Check sheet for the modelled part. Datum: model origin and axes. Units: mm. A direction names the side the tool comes from. Round coordinates to 2 decimals unless told otherwise and drop trailing zeros. Loops run counter-clockwise (first coordinate to the right, second up) from the corner with the lowest first, then second, coordinate; pieces in that order, holes last. Notation, with made-up numbers: (18, 27.5) - (52, 27.5) arc R19 ccw to (52, 44.5) - close; hole circle Ø6 at (-27.5, -11). An arc over 180 degrees is marked (long way). Return JSON: item names as keys, results as strings.
from build123d import *

# Parameters (mm, degrees)
SKETCH1_R           = 41
BOSS_EXTRUDE1_DEPTH = 6
BOSS_EXTRUDE2_DEPTH = 8
BOSS_EXTRUDE3_DEPTH = 7
SKETCH4_W           = 40.6
SKETCH4_H           = 20.7
CUT_EXTRUDE1_DEPTH  = 7
SKETCH5_R           = 9.55
CUT_EXTRUDE2_DEPTH  = 6.2
SKETCH6_R           = 7
CUT_EXTRUDE3_DEPTH  = 8
SKETCH7_R           = 11
SKETCH7_R_2         = 1.7
CUT_EXTRUDE4_DEPTH  = 6
SKETCH8_R           = 3.25
CUT_EXTRUDE6_DEPTH  = 3.3
SKETCH10_R          = 2.1
CUT_EXTRUDE8_DEPTH  = 5.5
FILLET1_R           = 3
CHAMFER1_SIZE       = 0.8
SKETCH11_W          = 7.2
SKETCH11_H          = 2
CUT_EXTRUDE9_DEPTH  = 2


with BuildPart() as part:
    # Sketch1 → Boss-Extrude1 (new body)
    with BuildSketch(Plane(origin=(0, 0, 0), x_dir=(1, 0, 0), z_dir=(0, 1, 0))):
        with Locations(Location((0, 0, 0), (0, 0, 270))):
            Circle(SKETCH1_R)
    extrude(amount=BOSS_EXTRUDE1_DEPTH)

    # Sketch2 → Boss-Extrude2 (add)
    with BuildSketch(Plane.XY.offset(-30)):
        with BuildLine():
            Line((-24, 0), (24, 0))
            Line((24, 0), (15.461253, 32.066997))
            ThreePointArc((15.461253, 32.066997), (0, 43.95000027), (-15.461253, 32.066997))
            Line((-15.461253, 32.066997), (-24, 0))
        make_face()
    extrude(amount=BOSS_EXTRUDE2_DEPTH)

    # Sketch3 → Boss-Extrude3 (add)
    with BuildSketch(Plane.XY.offset(22)):
        with BuildLine():
            Line((-40, 0), (20, 0))
            Line((20, 0), (20, 33))
            ThreePointArc((20, 33), (17.071067812, 40.071067812), (10, 43))
            Line((10, 43), (-30, 43))
            ThreePointArc((-30, 43), (-37.071067812, 40.071067812), (-40, 33))
            Line((-40, 33), (-40, 0))
        make_face()
    extrude(amount=BOSS_EXTRUDE3_DEPTH)

    # Sketch4 → Cut-Extrude1 (cut)
    with BuildSketch(Plane.XY.offset(22)):
        with Locations((-10.1, 28.05)):
            Rectangle(SKETCH4_W, SKETCH4_H)
    extrude(amount=CUT_EXTRUDE1_DEPTH, mode=Mode.SUBTRACT)

    # Sketch5 → Cut-Extrude2 (cut)
    with BuildSketch(Plane.XY.offset(-30)):
        with Locations(Location((0, 27.95, 0), (0, 0, 180))):
            Circle(SKETCH5_R)
    extrude(amount=CUT_EXTRUDE2_DEPTH, mode=Mode.SUBTRACT)

    # Sketch6 → Cut-Extrude3 (cut)
    with BuildSketch(Plane.XY.offset(-30)):
        with Locations((0, 27.95)):
            Circle(SKETCH6_R)
    extrude(amount=CUT_EXTRUDE3_DEPTH, mode=Mode.SUBTRACT)

    # Sketch7 → Cut-Extrude4 (cut)
    with BuildSketch(Plane(origin=(0, 0, 0), x_dir=(1, 0, 0), z_dir=(0, 1, 0))):
        with Locations(Location((0, 0, 0), (0, 0, 270))):
            Circle(SKETCH7_R)
        with Locations(Location((30, 15, 0), (0, 0, 270))):
            Circle(SKETCH7_R_2)
        with Locations(Location((30, -15, 0), (0, 0, 270))):
            Circle(SKETCH7_R_2)
        with Locations(Location((-30, 15, 0), (0, 0, 270))):
            Circle(SKETCH7_R_2)
        with Locations(Location((-30, -15, 0), (0, 0, 270))):
            Circle(SKETCH7_R_2)
    extrude(amount=CUT_EXTRUDE4_DEPTH, mode=Mode.SUBTRACT)

    # Sketch8 → Cut-Extrude6 (cut)
    with BuildSketch(Plane(origin=(0, 6, 0), x_dir=(1, 0, 0), z_dir=(0, 1, 0))):
        with Locations(Location((30, 15, 0), (0, 0, 270))):
            Circle(SKETCH8_R)
        with Locations(Location((30, -15, 0), (0, 0, 270))):
            Circle(SKETCH8_R)
        with Locations(Location((-30, 15, 0), (0, 0, 270))):
            Circle(SKETCH8_R)
        with Locations(Location((-30, -15, 0), (0, 0, 270))):
            Circle(SKETCH8_R)
    extrude(amount=-CUT_EXTRUDE6_DEPTH, mode=Mode.SUBTRACT)

    # Sketch10 → Cut-Extrude8 (cut)
    with BuildSketch(Plane.XY.offset(29)):
        with Locations((-34.811, 23.025)):
            Circle(SKETCH10_R)
        with Locations((-34.811, 32.875)):
            Circle(SKETCH10_R)
        with Locations((14.611, 23.025)):
            Circle(SKETCH10_R)
        with Locations((14.611, 32.875)):
            Circle(SKETCH10_R)
    extrude(amount=-CUT_EXTRUDE8_DEPTH, mode=Mode.SUBTRACT)

    # Fillet1
    fillet1_edges = [part.edges().sort_by_distance(p)[0] for p in [
        (0, 6, -22),
        (-7.298843892, 6, 22),
    ]]
    fillet(fillet1_edges, radius=FILLET1_R)

    # Chamfer1
    chamfer1_edges = [part.edges().sort_by_distance(p)[0] for p in [
        (-30, 0, 13.3),
        (-30, 0, -16.7),
        (30, 0, 13.3),
        (30, 0, -16.7),
    ]]
    chamfer(chamfer1_edges, length=CHAMFER1_SIZE)

    # Sketch11 → Cut-Extrude9 (cut)
    with BuildSketch(Plane.XY.offset(29)):
        with Locations((-33.8, 27.95)):
            Rectangle(SKETCH11_W, SKETCH11_H)
        with Locations((13.6, 27.95)):
            Rectangle(SKETCH11_W, SKETCH11_H)
    extrude(amount=-CUT_EXTRUDE9_DEPTH, mode=Mode.SUBTRACT)


solid = part.part
Q1. Draft check along X on faces 5 (the face through (17.15, 39.99, 25.45)), 6 (the face through (9, 0, 9)), 7 (the face through (26.827, 4.373, -15.705)). Enter one of: released by +X, released by -X, zero draft, split by the parting line, or undercut.
Answer key:
{"face 5": "released by +X", "face 6": "zero draft", "face 7": "undercut"}
Q2. Depth check by flat-ended pin: P1, Ø1, axis at y = 8.5, z = 22.5, coming from the +X side; P2, Ø5.5, axis at y = 13, z = 24.5, coming from the -X side; P3, Ø7.5, axis at x = -20, z = 25, coming from the +Y side; P4, Ø5, axis at y = 29, z = 18, coming from the -X side. Enter the tip coordinate at first touch or a pass-through.
Answer key:
{"P1": "stops at x = 20", "P2": "stops at x = -40", "P3": "stops at y = 43", "P4": "passes through"}
Q3. Sectioned sample at C-C (z = 0.5). Enter the section's corners in (x, y).
Answer key:
{"outline": "(-41, 0) - (-10.99, 0) - (-10.99, 6) - (-41, 6) - close; (10.99, 0) - (41, 0) - (41, 6) - (10.99, 6) - close"}
Q4. Tool access check on faces 1 (the face through (-31.4, 2.7, 16.4)), 2 (the face through (0, 19, -22)), 3 (the face through (-30.4, 28, 25)), 4 (the face through (10.2, 28, 25)). Record the directions out of +Z, -Z, +X, -X, +Y, -Y that give a thin tool (end or side, any length) a straight path to the whole face; none if there is none.
Answer key:
{"face 1": "+Y", "face 2": "+X, -X, +Y", "face 3": "+Z, -Z", "face 4": "+Z"}
Q5. Sectioned sample at D-D (x = 30). Enter the section's corners in (y, z), plus the area to 3 significant figures.
Answer key:
{"outline": "(0, -27.95) - (6, -27.95) - (6, -18.25) - (2.7, -18.25) - (2.7, -16.7) - (0.8, -16.7) - (0, -17.5) - close; (0, -12.5) - (0.8, -13.3) - (2.7, -13.3) - (2.7, -11.75) - (6, -11.75) - (6, 11.75) - (2.7, 11.75) - (2.7, 13.3) - (0.8, 13.3) - (0, 12.5) - close; (0, 17.5) - (0.8, 16.7) - (2.7, 16.7) - (2.7, 18.25) - (6, 18.25) - (6, 27.95) - (0, 27.95) - close", "area": "273 mm²"}
Q6. Sectioned sample at B-B (y = 16). Enter the section's corners in (x, z), plus the area to 3 significant figures.
Answer key:
{"outline": "(-40, 22) - (20, 22) - (20, 29) - (-40, 29) - close; (-19.74, -30) - (19.74, -30) - (19.74, -22) - (-19.74, -22) - close", "area": "736 mm²"}
Q7. Scan lines: probe 1 along X at (y, z) = (3, 15); probe 2 along X at (y, z) = (4, 0); probe 3 along Y at (x, z) = (-12.5, 28). Record each from-to range of solid material in increasing order. Write a range as [from, to].
Answer key:
{"probe 1": "x = [-38.16, -33.25], [-26.75, 26.75], [33.25, 38.16]", "probe 2": "x = [-41, -11], [11, 41]", "probe 3": "y = [0, 17.7], [38.4, 43]"}
Q8. Sectioned sample at A-A (x = 0). State how many separate pieces and enclosed holes the cut face has, plus the area to 3 significant figures.
Answer key:
{"separate pieces": "4", "enclosed holes": "0", "area": "638 mm²"}
